```python
from build123d import *

# Parameters (mm, degrees)
F0_R     = 125
F1_DEPTH = 10


# Not quite as in the source:
# - a feature names something its author has since deleted; it is built from what else it names


with BuildPart() as f1:
    # F0 (on Front) → F1 (new body)
    with BuildSketch(Plane.XZ):
        with BuildLine():
            ThreePointArc((0, -618.6190456596), (397.429722157, -420.8611796621), (538.6190456596, 0))
            ThreePointArc((538.6190456596, 0), (364.2926371672, 340.8611796621), (0, 458.6190456596))
            ThreePointArc((0, 458.6190456596), (-284.2926371672, 307.7240946723), (-378.6190456596, 0))
            ThreePointArc((-378.6190456596, 0), (-338.9932719851, -123.9081492515), (-255.845498181, -223.9575325662))
            Line((-255.845498181, -223.9575325662), (-248.8807463186, -229.5026751274))
            ThreePointArc((-248.8807463186, -229.5026751274), (-232.823383589, -285.1142187928), (-280.0241173048, -318.6190456596))
            Line((-280.0241173048, -318.6190456596), (-400, -318.6190456596))
            Line((-400, -318.6190456596), (-400, -618.6190456596))
            Line((-400, -618.6190456596), (0, -618.6190456596))
        make_face()
        Circle(F0_R, mode=Mode.SUBTRACT)
    extrude(amount=F1_DEPTH)


solid = f1.part
```
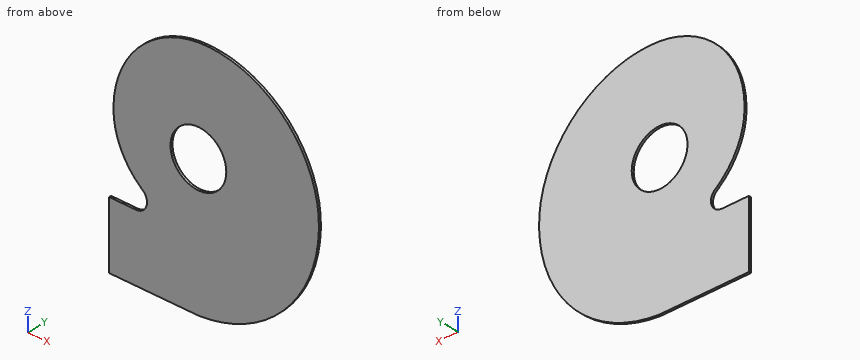
Could you check a few things on this model? Use its own coordinates, in mm. Round coordinates to 2 decimals unless told otherwise and drop trailing zeros. Loops run counter-clockwise (first coordinate to the right, second up) from the corner with the lowest first, then second, coordinate; pieces in that order, holes last. Notation, with made-up numbers: (-26.75, 88) - (18.25, 88) arc R22 cw to (18.25, 115) - close; hole circle Ø9 at (68.5, -33.5). An arc over 180 degrees is marked (long way). Answer in a Markdown table with one row per item. Add a question column.
(1) If we section it at C-C (z = 88.5): Please give me the cut outline in (x, y).
(2) If we section it at A-A (x = -53): Please give me the cut outline in (y, z), plus the area to 3 significant figures.
(3) I need wall thicknesses on line 1 along Z through (x, y) = (-40, -2.75); line 2 along Z through (x, y) = (-25, -3.5); line 3 along X through (y, z) = (-6, 110). Which ranges of each line are inside material? Lowest first, please.
(4) I'm going to push flat-ended pins straight in: pin 1 (5 mm diameter, centred on x = -332, y = -3, fed in from +Z); pin 2 (1 mm diameter, centred on x = 106.5, z = -224.5, fed in from +Y); pin 3 (1 mm diameter, centred on y = -2.5, z = 183, fed in from -X). Where does each tip first touch, or does it pass through?
(5) If we section it at D-D (x = 370): Please give me the cut outline in (y, z), plus the area to 3 significant figures.
(6) If we section it at B-B (y = -2): Please give me the cut outline in (x, z), plus the area to 3 significant figures.
Model answer:
| question | item | result |
|---|---|---|
| 1 | outline | (-377.72, -10) - (-88.28, -10) - (-88.28, 0) - (-377.72, 0) - close; (88.28, -10) - (523.43, -10) - (523.43, 0) - (88.28, 0) - close |
| 2 | outline | (-10, -618.62) - (0, -618.62) - (0, -113.21) - (-10, -113.21) - close; (-10, 113.21) - (0, 113.21) - (0, 450.11) - (-10, 450.11) - close |
| 2 | area | 8,420 mm² |
| 3 | line 1 | z = -618.62 to -118.43, 118.43 to 452.85 |
| 3 | line 2 | z = -618.62 to -122.47, 122.47 to 455.47 |
| 3 | line 3 | x = -374.66 to -59.37, 59.37 to 517.2 |
| 4 | pin 1 | stops at z = 240.78 |
| 4 | pin 2 | stops at y = 0 |
| 4 | pin 3 | stops at x = -355.65 |
| 5 | outline | (-10, -450.24) - (0, -450.24) - (0, 335.93) - (-10, 335.93) - close |
| 5 | area | 7,860 mm² |
| 6 | outline | (-400, -618.62) - (0, -618.62) arc R580 ccw to (538.62, 0) arc R500.22 ccw to (0, 458.62) arc R420.53 ccw to (-378.62, 0) arc R340.97 ccw to (-255.85, -223.96) - (-248.88, -229.5) arc R50 cw to (-280.02, -318.62) - (-400, -318.62) - close; hole circle Ø250 at (0, 0) |
| 6 | area | 764,000 mm² |
